```python
from build123d import *

# Parameters (mm, degrees)
BOX001_W               = 0.8
BOX001_H               = 0.8
BOX001_DEPTH           = 0.5
CHAMFER_SIZE           = 0.3
BOX_W                  = 10
BOX_H                  = 0.4
BOX_DEPTH              = 0.4
EXTRUDE001_DEPTH       = 1.3
FILLET_R               = 0.2
CUT005_PLACEMENT_ANGLE = 180
SKETCH_W               = 6.5
SKETCH_H               = 4.58
EXTRUDE_DEPTH          = 0.25
SKETCH001_W            = 6.1
SKETCH001_H            = 4.18


with BuildPart() as chamfer_body:
    # Box001 → Box001 (new body)
    with BuildSketch(Plane(origin=(-2.9, -0.2, -2), x_dir=(1, 0, 0), z_dir=(0, 0, 1))):
        with Locations((0.4, 0.4)):
            Rectangle(BOX001_W, BOX001_H)
    extrude(amount=BOX001_DEPTH)

    # Chamfer
    chamfer_edges = [chamfer_body.edges().sort_by_distance(p)[0] for p in [
        (-2.1, 0.6, -1.75),
    ]]
    chamfer(chamfer_edges, length=CHAMFER_SIZE)


with BuildPart() as chamfer_body_1:
    # Chamfer placement: moved
    add(chamfer_body.part.moved(Location((0.1, -0.1, 0))))


with BuildPart() as part_mirroring001:
    # Part__Mirroring001: instance of Chamfer body
    add(chamfer_body_1.part.mirror(Plane(origin=(0, 0.85, 0), x_dir=(1, 0, 0), z_dir=(0, 1, 0))))


with BuildPart() as part_mirroring002:
    # Part__Mirroring002: instance of Part__Mirroring001
    add(part_mirroring001.part.mirror(Plane(origin=(3.25, 0, 0), x_dir=(0, -1, 0), z_dir=(1, 0, 0))))


with BuildPart() as part_mirroring003:
    # Part__Mirroring003: instance of Part__Mirroring002
    add(part_mirroring002.part.mirror(Plane(origin=(0, 0.85, 0), x_dir=(1, 0, 0), z_dir=(0, 1, 0))))


with BuildPart() as cube:
    # Box → Box (new body)
    with BuildSketch(Plane(origin=(-1.5, 0.2, -0.3), x_dir=(1, 0, 0), z_dir=(0, 0, 1))):
        with Locations((5, 0.2)):
            Rectangle(BOX_W, BOX_H)
    extrude(amount=BOX_DEPTH)


with BuildPart() as cut003:
    # Sketch002 → Extrude001 (new body)
    with BuildSketch(Plane.XZ.offset(-0.2)):
        Polygon((-2.65, -1.875), (-1.83, -1.875), (-0.5, -0.05), (7, -0.05), (8.33, -1.875), (9.15, -1.875), (9.15, -1.775), (8.39, -1.775), (7.06, 0.05), (-0.56, 0.05), (-1.89, -1.775), (-2.65, -1.775), align=None)
    extrude(amount=EXTRUDE001_DEPTH)


with BuildPart() as cut003_1:
    # Extrude001 placement: moved
    add(cut003.part.moved(Location((0, 1.3, 0))))

    # Fillet
    fillet_edges = [cut003_1.edges().sort_by_distance(p)[0] for p in [
        (-1.83, 0.85, -1.875),
        (-0.5, 0.85, -0.05),
        (7, 0.85, -0.05),
        (8.33, 0.85, -1.875),
        (8.39, 0.85, -1.775),
        (7.06, 0.85, 0.05),
        (-0.56, 0.85, 0.05),
        (-1.89, 0.85, -1.775),
    ]]
    fillet(fillet_edges, radius=FILLET_R)

    # Cut: cut Cube
    add(cube.part, mode=Mode.SUBTRACT)

    # Cut001: cut Chamfer body
    add(chamfer_body_1.part, mode=Mode.SUBTRACT)

    # Cut002: cut Part__Mirroring001
    add(part_mirroring001.part, mode=Mode.SUBTRACT)

    # Cut003: cut Part__Mirroring002
    add(part_mirroring002.part, mode=Mode.SUBTRACT)


with BuildPart() as legs001:
    # Cut004 base: copy of Cut003
    add(cut003_1.part)

    # Cut004: cut Part__Mirroring003
    add(part_mirroring003.part, mode=Mode.SUBTRACT)


with BuildPart() as legs001_1:
    # Cut004 placement: moved
    add(legs001.part.moved(Location((0, 0.17, 0))))


with BuildPart() as legs002:
    # Cut005 base: copy of Cut003
    add(cut003_1.part)

    # Cut005: cut Part__Mirroring003
    add(part_mirroring003.part, mode=Mode.SUBTRACT)


with BuildPart() as legs002_1:
    # Cut005 placement: moved
    add(legs002.part.moved(Location((6.5, 4.41, 0))).rotate(Axis((6.5, 4.41, 0), (0, 0, 1)), CUT005_PLACEMENT_ANGLE))


with BuildPart() as extrude_body:
    # Sketch → Extrude (new body)
    with BuildSketch(Plane.XY.offset(0.125)):
        with Locations((3.25, 2.29)):
            Rectangle(SKETCH_W, SKETCH_H)
    extrude(amount=-EXTRUDE_DEPTH)


with BuildPart() as loft_body:
    # Sketch → Loft section 0
    with BuildSketch(Plane.XY.offset(0.125)):
        with Locations((3.25, 2.29)):
            Rectangle(SKETCH_W, SKETCH_H)
    # Sketch001 → Loft section 1
    with BuildSketch(Plane.XY.offset(1.625)):
        with Locations((3.25, 2.29)):
            Rectangle(SKETCH001_W, SKETCH001_H)
    loft()


with BuildPart() as part_mirroring:
    # Part__Mirroring: instance of Loft body
    add(loft_body.part.mirror(Plane(origin=(3.25, 2.29, 0), x_dir=(0, 1, 0), z_dir=(0, 0, 1))))


with BuildPart() as fusion001:
    # Fusion base: copy of Loft body
    add(loft_body.part)

    # Fusion: union Extrude body, Part__Mirroring
    add(extrude_body.part)
    add(part_mirroring.part)

    # Fusion001: union Legs001, Legs002
    add(legs001_1.part)
    add(legs002_1.part)


solid = fusion001.part
```
The model under review builds one solid part; all positions refer to its coordinate system, in mm. Round coordinates to 2 decimals unless told otherwise and drop trailing zeros. Write each loop counter-clockwise with the first axis right and the second up, starting at its lowest first coordinate (ties: lowest second). Pieces come first, ordered by that corner, then holes. Notation, with made-up numbers: (-38, -38) - (15, -38) arc R17 ccw to (15, -26) - close; hole circle Ø11 at (87.5, 87.25). An arc over 180 degrees is marked (long way). One line per question, with ' | ' between items.
Item 1: For P1, Ø1.5, axis at y = 4, z = 0, coming from the -X side; P2, Ø1.4, axis at x = 8, z = -1, coming from the +Y side; P3, Ø1, axis at x = -1, z = -1, coming from the -Y side, all flat-tipped, find the tip position at first contact; note any pin that passes through.
Resolved:
P1: stops at x = -1.14 | P2: stops at y = 4.21 | P3: stops at y = 0.37
Item 2: Add section B-B, the plane z = -1.15. State how many separate pieces and enclosed holes the cut face has, then the cut area to 3 significant figures.
Resolved:
separate pieces: 5 | enclosed holes: 0 | area: 27.5 mm2
Item 3: The part is to be moulded in two halves that separate along X. For faces 1 (the face through (3, 2, -1.625)), 2 (the face through (3, 2, 1.625)), say which applies: pulls with the +X half, pulls with the -X half, needs draft (parallel to the pull), parting line crosses it, or undercut.
Resolved:
face 1: undercut | face 2: needs draft
Item 4: Add section A-A, the plane x = 8. Give the boundary of the cut face in (y, z).
Resolved:
outline: (0.37, -1.42) - (1.67, -1.42) - (1.67, -1.24) - (0.37, -1.24) - close; (2.91, -1.42) - (4.21, -1.42) - (4.21, -1.24) - (2.91, -1.24) - close
Item 5: To check wall thickness, follow probe 1 along Z at (x, y) = (2.75, 2.25) (3 decimals); probe 2 along Y at (x, z) = (3.25, 0.5); probe 3 along Y at (x, z) = (2.5, -0.4). State the ranges of each line that lie inside material, in increasing order.
Resolved:
probe 1: z = -1.625 to 1.625 | probe 2: y = 0.05 to 4.53 | probe 3: y = 0.04 to 4.54
